```python
from build123d import *

# Parameters (mm, degrees)
SKETCH1_W           = 3.175
SKETCH1_H           = 9.525
SKETCH1_W_2         = 31.75
SKETCH1_H_2         = 47.625
SKETCH1_R           = 9.525
BOSS_EXTRUDE1_DEPTH = 3.175


with BuildPart() as part:
    # Sketch1 → Boss-Extrude1 (new body)
    # profile 1 of 5: a face of its own
    with BuildSketch(Plane.XY):
        with Locations((-17.4625, 12.7)):
            Rectangle(SKETCH1_W, SKETCH1_H)
    # profile 2 of 5: a face of its own
    with BuildSketch(Plane.XY):
        Rectangle(SKETCH1_W_2, SKETCH1_H_2)
        Circle(SKETCH1_R, mode=Mode.SUBTRACT)
    # profile 3 of 5: a face of its own
    with BuildSketch(Plane.XY):
        with Locations((-17.4625, -12.7)):
            Rectangle(SKETCH1_W, SKETCH1_H)
    # profile 4 of 5: a face of its own
    with BuildSketch(Plane.XY):
        with Locations((17.4625, 12.7)):
            Rectangle(SKETCH1_W, SKETCH1_H)
    # profile 5 of 5: a face of its own
    with BuildSketch(Plane.XY):
        with Locations((17.4625, -12.7)):
            Rectangle(SKETCH1_W, SKETCH1_H)
    extrude(amount=BOSS_EXTRUDE1_DEPTH)


solid = part.part
```
The listing builds one solid part. Answer for the finished solid, in the listing's coordinates (mm). A direction names the side the tool comes from. Round coordinates to 2 decimals unless told otherwise and drop trailing zeros. Loops run counter-clockwise (first coordinate to the right, second up) from the corner with the lowest first, then second, coordinate; pieces in that order, holes last.
Q1. Given pin 1 Ø1.6 at (x, z) = (-17.5, 1) entering from -Y; pin 2 Ø1.6 at (x, z) = (18, 1.5) entering from +Y; pin 3 Ø1 at (y, z) = (-22, 2) entering from -X (3 decimals), each flat-ended and moving along its own axis, determine where each tip first touches the part or whether it passes through.
Q2. Find the intervals of material crossed by line 1 (Y direction, x = 17.5, z = 0.9); line 2 (Y direction, x = 0, z = 1.5) (1 decimal); line 3 (X direction, y = -5, z = 1.6) (3 decimals), in increasing order.
Q3. Section A-A, the plane x = 0 is taken. Determine the outline of the cut face in (y, z) (1 decimal), then the cut area to 3 significant figures.
Q4. Which of the six approach directions +Z, -Z, +X, -X, +Y, -Y give full straight-line access (tool end or side, diameter ignored) to faces 4 (the face through (17, -17.462, 2)), 5 (the face through (15.875, 21, 2)), 6 (the face through (-15.875, -21, 2)), 7 (the face through (17, 7.937, 2)), 8 (the face through (-15.875, 21, 2))?
Q5. Section D-D, the plane y = 18 is taken. Determine the outline of the cut face in (x, z) (3 decimals), then the cut area to 3 significant figures.
Q6. For a pull along Y with two mould halves and no side action, classify faces 1 (the face through (-17, -17.462, 2)), 2 (the face through (-19.05, -13, 2)), 3 (the face through (-17, 7.937, 2)) as released by +Y, released by -Y, zero draft, split by the parting line, or undercut.
Q7. Section C-C, the plane y = 6 is taken. Determine the outline of the cut face in (x, z) (3 decimals), then the cut area to 3 significant figures.
Completed:
1. pin 1: stops at y = -17.46
1. pin 2: stops at y = 17.46
1. pin 3: stops at x = -15.875
2. line 1: y = -17.46 to -7.94, 7.94 to 17.46
2. line 2: y = -23.8 to -9.5, 9.5 to 23.8
2. line 3: x = -15.875 to -8.107, 8.107 to 15.875
3. outline: (-23.8, 0) - (-9.5, 0) - (-9.5, 3.2) - (-23.8, 3.2) - close; (9.5, 0) - (23.8, 0) - (23.8, 3.2) - (9.5, 3.2) - close
3. area: 90.7 mm2
4. face 4: +Z, -Z, +X, -Y
4. face 5: +Z, -Z, +X, +Y
4. face 6: +Z, -Z, -X, -Y
4. face 7: +Z, -Z, +X
4. face 8: +Z, -Z, -X, +Y
5. outline: (-15.875, 0) - (15.875, 0) - (15.875, 3.175) - (-15.875, 3.175) - close
5. area: 101 mm2
6. face 1: released by -Y
6. face 2: zero draft
6. face 3: undercut
7. outline: (-15.875, 0) - (-7.398, 0) - (-7.398, 3.175) - (-15.875, 3.175) - close; (7.398, 0) - (15.875, 0) - (15.875, 3.175) - (7.398, 3.175) - close
7. area: 53.8 mm2
